Design review of the part shown in the three views and the two pictorial views. Dimensions are in mm from the part's minimum x, y and z. Give positions to 0.01 mm unless a question says otherwise; leave off trailing zeros. Loops run counter-clockwise (first coordinate to the right, second up) from the corner with the lowest first, then second, coordinate; pieces in that order, holes last. Notation, with made-up numbers: (-4.75, -38) - (16.25, -38) arc R21 cw to (16.25, -18) - close; hole circle Ø11 at (18.5, 71). An arc over 180 degrees is marked (long way). Answer as a JSON object with one key per item and string values.
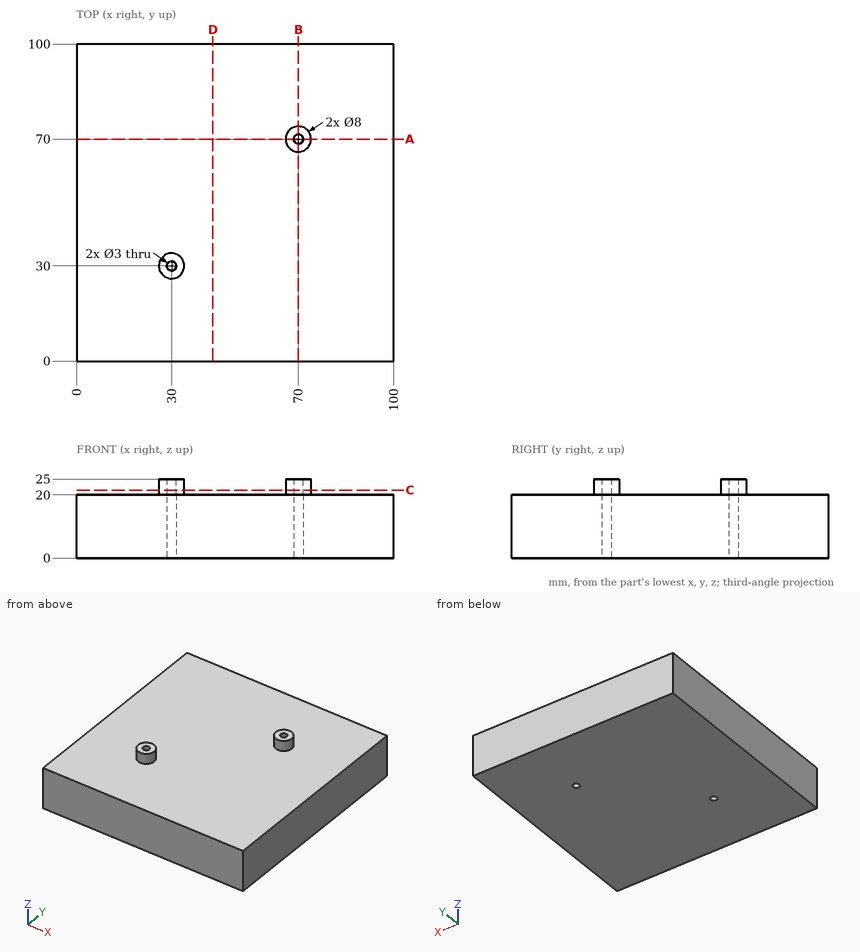
Q1. To check wall thickness, follow probe 1 along X at (y, z) = (70, 13.75); probe 2 along Y at (x, z) = (30, 15). State the ranges of each line that lie inside material, in increasing order. Write a range as [from, to].
Results:
{"probe 1": "x = [0, 68.5], [71.5, 100]", "probe 2": "y = [0, 28.5], [31.5, 100]"}
Q2. Consider section A-A, the plane y = 70. State the section outline as (x, z) points.
Results:
{"outline": "(0, 0) - (68.5, 0) - (68.5, 25) - (66, 25) - (66, 20) - (0, 20) - close; (71.5, 0) - (100, 0) - (100, 20) - (74, 20) - (74, 25) - (71.5, 25) - close"}
Q3. Consider section C-C, the plane z = 21.5. State the section outline as (x, y) points.
Results:
{"outline": "circle Ø8 at (30, 30); circle Ø8 at (70, 70); hole circle Ø3 at (30, 30); hole circle Ø3 at (70, 70)"}
Q4. Clearance check with flat-ended pins moving along their axes: pin 1 Ø3.5 at (x, y) = (70, 70) entering from -Z; pin 2 Ø12 at (x, y) = (41, 65) entering from +Z. State where each tip first meets the part, or that it passes through.
Results:
{"pin 1": "stops at z = 0", "pin 2": "stops at z = 20"}
Q5. Consider section D-D, the plane x = 43. State the section outline as (y, z) points.
Results:
{"outline": "(0, 0) - (100, 0) - (100, 20) - (0, 20) - close"}
